CAD build for the part. Positions are in the model's coordinates, mm. A direction names the side the tool comes from. Give positions to 0.01 mm unless a question says otherwise; leave off trailing zeros. Write each loop counter-clockwise with the first axis right and the second up, starting at its lowest first coordinate (ties: lowest second). Pieces come first, ordered by that corner, then holes. Notation, with made-up numbers: (-26, 27) -> (8, 27) arc R17 ccw to (8, 37) -> close; hole circle Ø6 at (24.5, 67.25). An arc over 180 degrees is marked (long way). Answer in a Markdown table with one row per item. Add a question column.
```python
from build123d import *

# Parameters (mm, degrees)
SKETCH1_W             = 25.4
SKETCH1_H             = 25.4
BOSS_EXTRUDE1_DEPTH   = 12.7
BOSS_EXTRUDE1_2_DEPTH = 12.7
BOSS_EXTRUDE2_DEPTH   = 25.4
SKETCH3_R             = 3.175
CUT_EXTRUDE1_DEPTH    = 100.190170884
FILLET1_R             = 12.7
BOSS_EXTRUDE3_DEPTH   = 76.2
SKETCH5_W             = 25.4
SKETCH5_H             = 50.8
CUT_EXTRUDE2_DEPTH    = 96.882897328


with BuildPart() as part:
    # Sketch1 → Boss-Extrude1 (new, symmetric)
    with BuildSketch(Plane.XY):
        with Locations((-12.7, 12.7)):
            Rectangle(SKETCH1_W, SKETCH1_H)
    extrude(amount=BOSS_EXTRUDE1_DEPTH, both=True)



with BuildPart() as body_2:
    # Sketch1 → Boss-Extrude1 2 (new, symmetric)
    with BuildSketch(Plane.XY):
        with Locations((38.1, 12.7)):
            Rectangle(SKETCH1_W, SKETCH1_H)
    extrude(amount=BOSS_EXTRUDE1_2_DEPTH, both=True)


with BuildPart() as part_1:
    add(part.part)

    add(body_2.part)  # Boss-Extrude2 merges body 2
    # Sketch2 → Boss-Extrude2 (add)
    with BuildSketch(Plane(origin=(0, 0, -12.7), x_dir=(-1, 0, 0), z_dir=(0, 0, -1))):
        Polygon((-50.8, 25.4), (-25.4, 50.8), (0, 50.8), (25.4, 25.4), (25.4, 0), (0, -25.4), (-25.4, -25.4), (-50.8, 0), align=None)
    extrude(amount=BOSS_EXTRUDE2_DEPTH)

    # Sketch3 → Cut-Extrude1 (cut, through all)
    with BuildSketch(Plane(origin=(50.8, 0, 0), x_dir=(0, 0, -1), z_dir=(1, 0, 0))):
        with Locations(Location((0, 12.7, 0), (0, 0, 90))):
            Circle(SKETCH3_R)
    extrude(amount=-CUT_EXTRUDE1_DEPTH, mode=Mode.SUBTRACT)

    # Fillet1
    fillet1_edges = [part_1.edges().sort_by_distance(p)[0] for p in [
        (38.1, 0, 12.7),
        (-12.7, 0, 12.7),
        (-12.7, 25.4, 12.7),
        (38.1, 25.4, 12.7),
    ]]
    fillet(fillet1_edges, radius=FILLET1_R - 0.0001)  # a hair under: the kernel refuses the full size

    # Sketch4 → Boss-Extrude3 (add)
    with BuildSketch(Plane(origin=(0, 50.8, 0), x_dir=(1, 0, 0), z_dir=(0, 1, 0))):
        with BuildLine():
            ThreePointArc((0, 50.8), (3.719743896, 41.819743862), (12.700000049, 38.1))
            ThreePointArc((12.700000049, 38.1), (21.680256138, 41.819743896), (25.4, 50.8))
            Line((25.4, 50.8), (15.875, 50.8))
            ThreePointArc((15.875, 50.8), (12.7, 47.625), (9.525, 50.8))
            Line((9.525, 50.8), (0, 50.8))
        make_face()
        with BuildLine():
            ThreePointArc((25.4, 50.8), (12.7, 63.5), (0, 50.8))
            Line((0, 50.8), (9.525, 50.8))
            ThreePointArc((9.525, 50.8), (12.7, 53.975), (15.875, 50.8))
            Line((15.875, 50.8), (25.4, 50.8))
        make_face()
        with BuildLine():
            Line((0, 50.8), (0, 38.1))
            Line((0, 38.1), (12.700000049, 38.1))
            ThreePointArc((12.700000049, 38.1), (3.719743896, 41.819743862), (0, 50.8))
        make_face()
        with BuildLine():
            ThreePointArc((25.4, 50.8), (21.680256138, 41.819743896), (12.700000049, 38.1))
            Line((12.700000049, 38.1), (25.4, 38.1))
            Line((25.4, 38.1), (25.4, 50.8))
        make_face()
    extrude(amount=-BOSS_EXTRUDE3_DEPTH)

    # Sketch5 → Cut-Extrude2 (cut, through all)
    with BuildSketch(Plane(origin=(25.4, 0, 0), x_dir=(0, 0, -1), z_dir=(1, 0, 0))):
        with Locations((50.8, 12.7)):
            Rectangle(SKETCH5_W, SKETCH5_H)
    extrude(amount=-CUT_EXTRUDE2_DEPTH, mode=Mode.SUBTRACT)


solid = part_1.part
```
Item 1: Which spindle directions (+Z, -Z, +X, -X, +Y, -Y) get a long thin tool onto all of the face, cutting with end or side? Do faces 4 (the face through (0, -19, -45)), 5 (the face through (0, 15, -3)), 6 (the face through (10, 38.1, -48)). Say none if no direction does.
Item 2: Mould opens along X. For faces 1 (the face through (12.29, -18.96, -47.65)), 2 (the face through (-13, 0, -6)), 3 (the face through (25.4, -19, -44)) say: released by +X, released by -X, zero draft, split by the parting line, or undercut.
Item 3: Slice it at D-D, the plane x = 12.7. List the corners of the cut face in (y, z) (3 decimals).
Item 4: Drop flat-ended pins along their axis: pin 1 Ø5 at (y, z) = (-12, -53.5) entering from +X; pin 2 Ø8 at (y, z) = (33, -31.5) entering from +X; pin 3 Ø12 at (x, z) = (32, -38) entering from +Y. Give the stop position or say it passes through.
Item 5: Probe L1, parallel to X at y = 6.5, z = -1.5; L2, parallel to Z at x = 43.25, y = 12.7 (3 decimals); L3, parallel to Z at x = 6, y = 14.5. List the from-to ranges inside material, lowest first. Write a range as from..to.
Item 6: Slice it at A-A, the plane z = -42. List the corners of the cut face in (x, y).
Item 7: Slice it at C-C, the plane y = -14.5. List the corners of the cut face in (x, z) (3 decimals).
Answer key:
| question | item | result |
|---|---|---|
| 1 | face 4 | -Z, -X, +Y, -Y |
| 1 | face 5 | +Z, +Y, -Y |
| 1 | face 6 | -Z, +X, -X |
| 2 | face 1 | undercut |
| 2 | face 2 | zero draft |
| 2 | face 3 | released by +X |
| 3 | outline | (-25.4, -63.5) -> (-12.7, -63.5) -> (-12.7, -53.975) -> (-25.4, -53.975) -> close; (-25.4, -47.625) -> (-12.7, -47.625) -> (-12.7, -38.1) -> (38.1, -38.1) -> (38.1, -47.625) -> (50.8, -47.625) -> (50.8, -12.7) -> (-25.4, -12.7) -> close; (38.1, -63.5) -> (50.8, -63.5) -> (50.8, -53.975) -> (38.1, -53.975) -> close |
| 4 | pin 1 | stops at x = 25.4 |
| 4 | pin 2 | stops at x = 47.2 |
| 4 | pin 3 | stops at y = 50.2 |
| 5 | L1 | x = -25.4..0, 25.4..50.8 |
| 5 | L2 | z = -38.1..-3.175, 3.175..12.7 |
| 5 | L3 | z = -38.1..-12.7 |
| 6 | outline | (0, -25.4) -> (25.4, -25.4) -> (25.4, -12.7) -> (0, -12.7) -> close; (0, 38.1) -> (25.4, 38.1) -> (25.4, 50.8) -> (0, 50.8) -> close |
| 7 | outline | (-10.9, -38.1) -> (0, -38.1) -> (0, -50.8) arc R12.7 ccw to (25.4, -50.8) -> (25.4, -38.1) -> (36.3, -38.1) -> (36.3, -12.7) -> (-10.9, -12.7) -> close; hole circle Ø6.35 at (12.7, -50.8) |
